from build123d import *

# Parameters (mm, degrees)
F0_R     = 12.7
F1_DEPTH = 3.175


with BuildPart() as f1:
    # F0 (on Top) → F1 (new body)
    with BuildSketch(Plane.XY):
        with BuildLine():
            ThreePointArc((-16.82951, -27.128529), (-7.628193, -26.097033), (0, -20.849283))
            ThreePointArc((0, -20.849283), (7.628193, -26.097033), (16.82951, -27.128529))
            ThreePointArc((16.82951, -27.128529), (22.225, -21.997045), (29.36674, -19.890155))
            ThreePointArc((29.36674, -19.890155), (30.785284, -17.773892), (31.90875, -15.487265))
            ThreePointArc((31.90875, -15.487265), (30.1625, -8.248892), (31.90875, -1.010519))
            ThreePointArc((31.90875, -1.010519), (26.41479, 6.442307), (18.056008, 10.424641))
            ThreePointArc((18.056008, 10.424641), (18.786597, 19.654725), (15.07924, 28.139047))
            ThreePointArc((15.07924, 28.139047), (7.9375, 30.245937), (2.54201, 35.377421))
            ThreePointArc((2.54201, 35.377421), (0, 35.547784), (-2.54201, 35.377421))
            ThreePointArc((-2.54201, 35.377421), (-7.9375, 30.245937), (-15.07924, 28.139047))
            ThreePointArc((-15.07924, 28.139047), (-18.786597, 19.654725), (-18.056008, 10.424641))
            ThreePointArc((-18.056008, 10.424641), (-26.41479, 6.442307), (-31.90875, -1.010519))
            ThreePointArc((-31.90875, -1.010519), (-30.1625, -8.248892), (-31.90875, -15.487265))
            ThreePointArc((-31.90875, -15.487265), (-30.785284, -17.773892), (-29.36674, -19.890155))
            ThreePointArc((-29.36674, -19.890155), (-22.225, -21.997045), (-16.82951, -27.128529))
        make_face()
        with Locations((-14.2875, -8.248892)):
            Circle(F0_R, mode=Mode.SUBTRACT)
        with Locations((14.2875, -8.248892)):
            Circle(F0_R, mode=Mode.SUBTRACT)
        with Locations((0, 16.497784)):
            Circle(F0_R, mode=Mode.SUBTRACT)
    extrude(amount=F1_DEPTH)


solid = f1.part
Read the model definition and answer for the solid it produces. Units are mm, in the model's axes. Coordinates: 2 decimals unless noted, no trailing zeros. Loops run counter-clockwise (first coordinate to the right, second up) from the corner with the lowest first, then second, coordinate; pieces in that order, holes last. Notation, with made-up numbers: (-14.5, -8.5) -> (44.5, -8.5) arc R22 ccw to (44.5, 25.5) -> close; hole circle Ø3 at (62, -38). An arc over 180 degrees is marked (long way). Write item = value, one per line. Start each with the question number.
1) The part is cut by section A-A, the plane x = -22. Determine the outline of the cut face in (y, z) (3 decimals).
2) The mould has two halves that part along Y. Classify faces 1 (the face through (8.029, 30.194, 1.565)), 2 (the face through (18.808, 19.526, 1.565)), 3 (the face through (30.77, -17.8, 1.57)): pulls with the +Y half, pulls with the -Y half, needs draft (parallel to the pull), parting line crosses it, or undercut.
3) Find the intervals of material crossed by L1, parallel to X at y = 3.5, z = 0.8; L2, parallel to Y at x = 5.5, z = 0.7; L3, parallel to X at y = -7, z = 2, in increasing order. Write a range as from..to.
4) The part is cut by section D-D, the plane z = 2.55. State how many separate pieces and enclosed holes the cut face has, plus the area to 3 significant figures.
5) The part is cut by section C-C, the plane y = 1. Determine the outline of the cut face in (x, z) (3 decimals).
6) The part is cut by section B-B, the plane y = 21. Determine the outline of the cut face in (x, z) (3 decimals).
Result:
q1.outline = (-22.129, 0) -> (-18.339, 0) -> (-18.339, 3.175) -> (-22.129, 3.175) -> close; (1.841, 0) -> (9.17, 0) -> (9.17, 3.175) -> (1.841, 3.175) -> close
q2.face_1 = pulls with the +Y half
q2.face_2 = undercut
q2.face_3 = pulls with the -Y half
q3.L1 = -29.28..-19.11, -9.47..9.47, 19.11..29.28
q3.L2 = -25.15..-17.42, 0.92..5.05, 27.95..31.98
q3.L3 = -30.21..-26.93, -1.65..1.65, 26.93..30.21
q4.separate_pieces = 1
q4.enclosed_holes = 3
q4.area = 1,250 mm²
q5.outline = (-30.942, 0) -> (-22.991, 0) -> (-22.991, 3.175) -> (-30.942, 3.175) -> close; (-5.584, 0) -> (5.584, 0) -> (5.584, 3.175) -> (-5.584, 3.175) -> close; (22.991, 0) -> (30.942, 0) -> (30.942, 3.175) -> (22.991, 3.175) -> close
q6.outline = (-18.51, 0) -> (-11.875, 0) -> (-11.875, 3.175) -> (-18.51, 3.175) -> close; (11.875, 0) -> (18.51, 0) -> (18.51, 3.175) -> (11.875, 3.175) -> close
